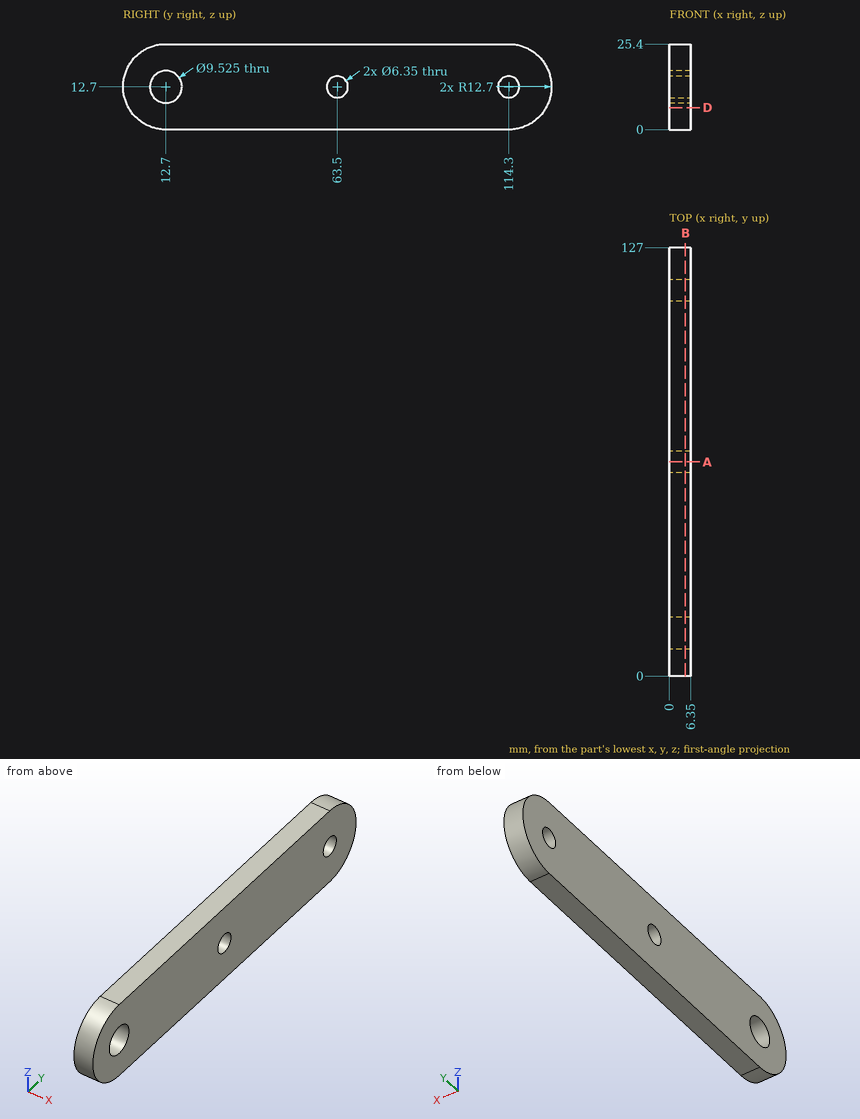
The drawing under review shows one solid part. Ordinate dimensions are in mm from its lowest x, y, z. Coordinates: 2 decimals unless noted, no trailing zeros. Order: outer loops, then holes, each group sorted by start corner. A loop starts at its lowest first (then second) coordinate and runs counter-clockwise, first axis right, second up. Notation, with made-up numbers: M 30,23 L 38,23 A24 cw 38,34 Z; hole C 46.25,-14 d2. An arc over 180 degrees is marked long. Use a Markdown table: item, result.
(1) Wall thickness on probe 1 along Y at (x, z) = (1.5, 12.7) (1 decimal); probe 2 along Y at (x, z) = (4.5, 15.5); probe 3 along Y at (x, z) = (4, 8.75): over which ranges is each line inside the solid? List them lowest first.
Worked answers:
| item | result |
|---|---|
| probe 1 | y = 0 to 7.9, 17.5 to 60.3, 66.7 to 111.1, 117.5 to 127 |
| probe 2 | y = 0.31 to 8.85, 16.55 to 62, 65 to 112.8, 115.8 to 126.69 |
| probe 3 | y = 0.63 to 10.04, 15.36 to 126.37 |
(2) For P1, Ø5.5, axis at y = 114.3, z = 12.7, coming from the -X side; P2, Ø1, axis at x = 1.5, z = 8.5, coming from the +Y side, all flat-tipped, find the tip position at first contact; note any pin that passes through.
Worked answers:
| item | result |
|---|---|
| P1 | passes through |
| P2 | stops at y = 126.45 |
(3) Add section A-A (y = 63.5). Give the boundary of the cut face in (x, z) (3 decimals).
Worked answers:
| item | result |
|---|---|
| outline | M 0,0 L 6.35,0 L 6.35,9.525 L 0,9.525 Z; M 0,15.875 L 6.35,15.875 L 6.35,25.4 L 0,25.4 Z |
(4) Add section D-D (z = 6.5). Give the boundary of the cut face in (x, y).
Worked answers:
| item | result |
|---|---|
| outline | M 0,1.62 L 6.35,1.62 L 6.35,125.38 L 0,125.38 Z |
(5) Add section B-B (x = 4.75). Count the separate pieces of the cut face and the enclosed holes in it, then the cut area to 3 significant figures.
Worked answers:
| item | result |
|---|---|
| separate pieces | 1 |
| enclosed holes | 3 |
| area | 2,950 mm2 |
